```python
from build123d import *

# Parameters (mm, degrees)
F0_W      = 66
F0_H      = 38
F1_DEPTH  = 2
F2_W      = 61.6
F2_H      = 33.6
F2_W_2    = 59.6
F2_H_2    = 31.6
F3_DEPTH  = 6.8
F4_R      = 2
F5_W      = 45
F5_H      = 35
F6_DEPTH  = 1
F7_R      = 1
F8_DEPTH  = 8.801
F9_W      = 4
F9_H      = 9.6
F10_DEPTH = 6.8
F11_R     = 1.5
F12_DEPTH = 35.801
F13_SIZE  = 1


with BuildPart() as f1:
    # F0 (on Top) → F1 (new body)
    with BuildSketch(Plane.XY):
        with Locations((33, -19)):
            Rectangle(F0_W, F0_H)
    extrude(amount=F1_DEPTH)

    # F2 (on face) → F3 (join)
    with BuildSketch(Plane.XY.offset(2)):
        with Locations((33, -19)):
            Rectangle(F2_W, F2_H)
        with Locations((33, -19)):
            Rectangle(F2_W_2, F2_H_2, mode=Mode.SUBTRACT)
    extrude(amount=F3_DEPTH)

    # F4
    f4_edges = [f1.edges().sort_by_distance(p)[0] for p in [
        (0, -38, 1),
        (0, 0, 1),
        (66, -38, 1),
        (66, 0, 1),
    ]]
    fillet(f4_edges, radius=F4_R)

    # F5 (on face) → F6 (cut)
    with BuildSketch(Plane(origin=(0, 0, 0), x_dir=(1, 0, 0), z_dir=(0, 0, -1))):
        with Locations((24.5, 19)):
            Rectangle(F5_W, F5_H)
    extrude(amount=-F6_DEPTH, mode=Mode.SUBTRACT)

    # F7 (on face) → F8 (cut, through all)
    with BuildSketch(Plane(origin=(0, 0, 0), x_dir=(1, 0, 0), z_dir=(0, 0, -1))):
        with Locations((9.5, 32.5)):
            Circle(F7_R)
        with Locations((39.5, 32.5)):
            Circle(F7_R)
    extrude(amount=-F8_DEPTH, mode=Mode.SUBTRACT)

    # F9 (on face) → F10 (join)
    with BuildSketch(Plane.XY.offset(2)):
        with Locations((5.2, -19)):
            Rectangle(F9_W, F9_H)
        with Locations((60.8, -19)):
            Rectangle(F9_W, F9_H)
    extrude(amount=F10_DEPTH)

    # F11 (on face) → F12 (cut, through all)
    with BuildSketch(Plane(origin=(0, -2.2, 0), x_dir=(-1, 0, 0), z_dir=(0, 1, 0))):
        with Locations((-61, 5)):
            Circle(F11_R)
        with Locations((-5, 5)):
            Circle(F11_R)
    extrude(amount=-F12_DEPTH, mode=Mode.SUBTRACT)

    # F13
    f13_edges = [f1.edges().sort_by_distance(p)[0] for p in [
        (2.2, -2.2, 5.4),
        (2.2, -35.8, 5.4),
        (63.8, -35.8, 5.4),
        (63.8, -2.2, 5.4),
    ]]
    chamfer(f13_edges, length=F13_SIZE)


solid = f1.part
```
Input: part model. Units: mm. Frame: model coordinates. A direction names the side the tool comes from. Round coordinates to 2 decimals unless told otherwise and drop trailing zeros. Loops run counter-clockwise (first coordinate to the right, second up) from the corner with the lowest first, then second, coordinate; pieces in that order, holes last. Notation, with made-up numbers: (20, 26) -> (57, 26) arc R29 ccw to (57, 60) -> close; hole circle Ø1 at (0.25, 27). An arc over 180 degrees is marked (long way). One line per item, written item: value.
(1) Section D-D (x = 39.5). Return the cut outline in (y, z).
Geometry check:
outline: (-38, 0) -> (-36.5, 0) -> (-36.5, 1) -> (-33.5, 1) -> (-33.5, 2) -> (-34.8, 2) -> (-34.8, 8.8) -> (-35.8, 8.8) -> (-35.8, 2) -> (-38, 2) -> close; (-31.5, 1) -> (-1.5, 1) -> (-1.5, 0) -> (0, 0) -> (0, 2) -> (-2.2, 2) -> (-2.2, 8.8) -> (-3.2, 8.8) -> (-3.2, 2) -> (-31.5, 2) -> close
(2) Section A-A (y = -32.5). Return the cut outline in (x, z), plus the area to 3 significant figures.
Geometry check:
outline: (0, 0) -> (2, 0) -> (2, 1) -> (8.5, 1) -> (8.5, 2) -> (3.2, 2) -> (3.2, 8.8) -> (2.2, 8.8) -> (2.2, 2) -> (0, 2) -> close; (10.5, 1) -> (38.5, 1) -> (38.5, 2) -> (10.5, 2) -> close; (40.5, 1) -> (47, 1) -> (47, 0) -> (66, 0) -> (66, 2) -> (63.8, 2) -> (63.8, 8.8) -> (62.8, 8.8) -> (62.8, 2) -> (40.5, 2) -> close
area: 96.6 mm2
(3) Pin query (flat end, axial travel): pin 1 (2.5 mm diameter, centred on x = 5, z = 5, fed in from +Y); pin 2 (1 mm diameter, centred on x = 42.5, y = -5.5, fed in from +Z); pin 3 (1 mm diameter, centred on y = -22.5, z = 3.5, fed in from -X); pin 4 (3.5 mm diameter, centred on y = -9, z = 7, fed in from +X). Return the tip coordinate at first contact, or that it passes through.
Geometry check:
pin 1: through
pin 2: z = 2
pin 3: x = 2.2
pin 4: x = 63.8
(4) Material intervals for line 1 (Z direction, x = 5, y = -18.5); line 2 (Y direction, x = 9.5, z = 1.65); line 3 (X direction, y = -32.5, z = 1.3), sorted ascending. Write a range as [from, to].
Geometry check:
line 1: [1, 3.5], [6.5, 8.8]
line 2: [-38, -33.5], [-31.5, 0]
line 3: [0, 8.5], [10.5, 38.5], [40.5, 66]
(5) Set-up query: faces 4 (the face through (33, -34.8, 5)), 5 (the face through (33, 0, 1)), 6 (the face through (33, -2.2, 5)). Return all of +Z, -Z, +X, -X, +Y, -Y with unobstructed straight access to the full face (end or side cutting, diameter ignored); none if empty.
Geometry check:
face 4: +Z
face 5: +Z, -Z, +X, -X, +Y
face 6: +Z, +X, -X, +Y
(6) Section B-B (y = -23). Return the cut outline in (x, z), plus the area to 3 significant figures.
Geometry check:
outline: (0, 0) -> (2, 0) -> (2, 1) -> (47, 1) -> (47, 0) -> (66, 0) -> (66, 2) -> (63.8, 2) -> (63.8, 8.8) -> (58.8, 8.8) -> (58.8, 2) -> (7.2, 2) -> (7.2, 8.8) -> (2.2, 8.8) -> (2.2, 2) -> (0, 2) -> close; hole circle Ø3 at (5, 5); hole circle Ø3 at (61, 5)
area: 141 mm2
(7) Mould query, pull axis Y, two halves, no side actions, for faces 1 (the face through (48, -16, 0)), 2 (the face through (0.57, -37.4, 1.01)), 3 (the face through (7, -23.8, 5)). Classes: pulls with the +Y half, pulls with the -Y half, needs draft (parallel to the pull), parting line crosses it, or undercut.
Geometry check:
face 1: needs draft
face 2: pulls with the -Y half
face 3: undercut
(8) Section C-C (x = 5). Give the number of separate pieces and of enclosed holes in the cut face, plus the area to 3 significant figures.
Geometry check:
separate pieces: 4
enclosed holes: 0
area: 85.1 mm2
